Here's the drawing with two shaded views (mm, measured from the low corner). I have some questions. A direction names the side the tool comes from. Round coordinates to 2 decimals unless told otherwise and drop trailing zeros. Order: outer loops, then holes, each group sorted by start corner. A loop starts at its lowest first (then second) coordinate and runs counter-clockwise, first axis right, second up. Notation, with made-up numbers: (-8.5, -38) - (37.5, -38) arc R29 cw to (37.5, -6) - close; hole circle Ø7 at (82.25, -32.5). An arc over 180 degrees is marked (long way). Return JSON: item names as keys, results as strings. Group by question number.
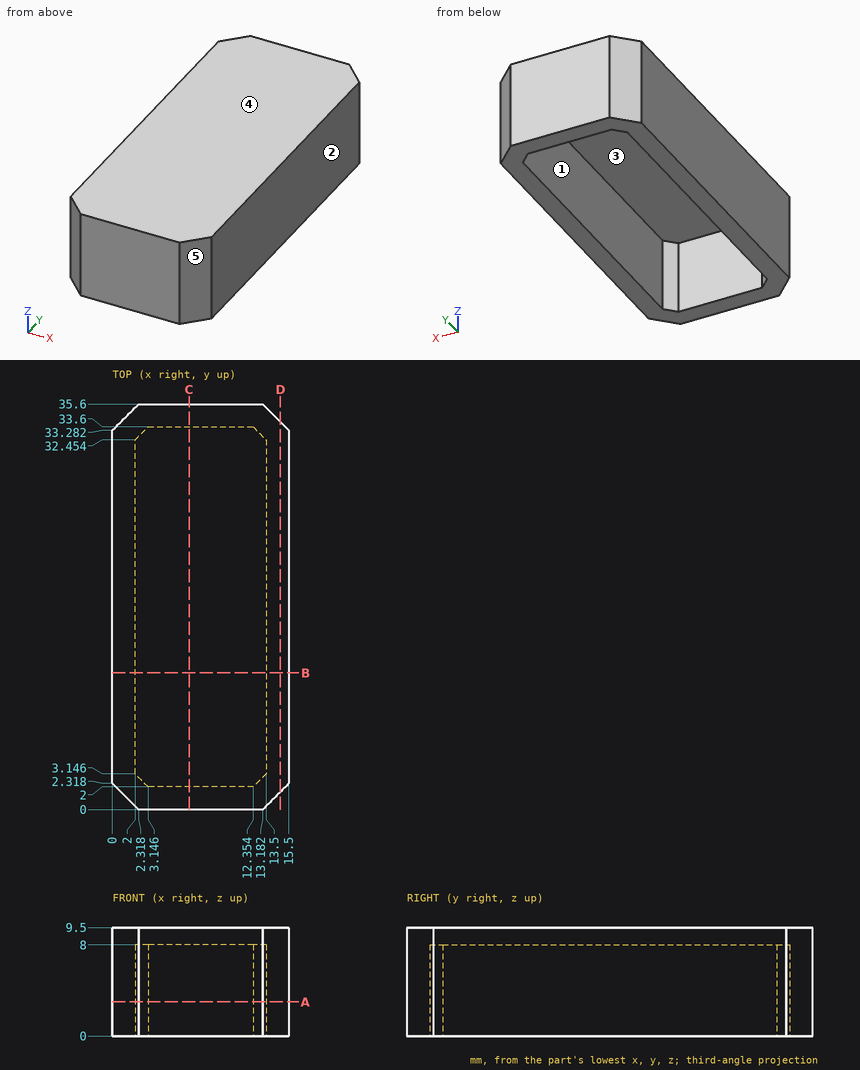
1) I want a section at D-D, the plane x = 14.75. List the corners of the cut face in (y, z) for me.
2) We'd pull the mould along X, two halves only. Please class the marked faces 3, 4 and 5: +X half, -X half, draft (parallel to the pull), parting line (faces both ways), or undercut.
3) Will this pin go through, and if not, where does the flat tip stop? pin 1 (1 mm diameter, centred on x = 10, y = 18, fed in from -Z).
4) I want a section at C-C, the plane x = 6.75. List the corners of the cut face in (y, z) for me.
5) I want a section at A-A, the plane z = 3. List the corners of the cut face in (x, y) for me, plus the area to 3 significant figures.
6) For the marked faces 1 and 2, which set-ups out of +Z, -Z, +X, -X, +Y, -Y let a thin tool reach every point of the face, with its end or its side?
7) If I drill on line 1 along X through (y, z) = (21, 3); line 2 along Y through (x, z) = (4.25, 6.5); line 3 along Z through (x, y) = (6.75, 32), over which ranges is the centre line in solid material (lowest first)? Write a range as from..to.
8) I want a section at B-B, the plane y = 12. List the corners of the cut face in (x, z) for me.
Outcome:
{
 "1": {"outline": "(1.57, 0) - (34.03, 0) - (34.03, 9.5) - (1.57, 9.5) - close"},
 "2": {"face 3": "undercut", "face 4": "draft", "face 5": "+X half"},
 "3": {"pin 1": "z = 8"},
 "4": {"outline": "(0, 0) - (2, 0) - (2, 8) - (33.6, 8) - (33.6, 0) - (35.6, 0) - (35.6, 9.5) - (0, 9.5) - close"},
 "5": {"outline": "(0, 2.32) - (2.32, 0) - (13.18, 0) - (15.5, 2.32) - (15.5, 33.28) - (13.18, 35.6) - (2.32, 35.6) - (0, 33.28) - close; hole (2, 3.15) - (3.15, 2) - (12.35, 2) - (13.5, 3.15) - (13.5, 32.45) - (12.35, 33.6) - (3.15, 33.6) - (2, 32.45) - close", "area": "180 mm^2"},
 "6": {"face 1": "-Z", "face 2": "+Z, -Z, +X, +Y, -Y"},
 "7": {"line 1": "0..2, 13.5..15.5", "line 2": "0..2, 33.6..35.6", "line 3": "8..9.5"},
 "8": {"outline": "(0, 0) - (2, 0) - (2, 8) - (13.5, 8) - (13.5, 0) - (15.5, 0) - (15.5, 9.5) - (0, 9.5) - close"}
}
